Input: part model. Units: mm. Frame: model coordinates. A direction names the side the tool comes from. Coordinates: 2 decimals unless noted, no trailing zeros. Loops run counter-clockwise (first coordinate to the right, second up) from the corner with the lowest first, then second, coordinate; pieces in that order, holes last. Notation, with made-up numbers: (22.5, 86) - (56.5, 86) arc R21 cw to (56.5, 110) - close; hole circle Ø9 at (65, 2). An arc over 180 degrees is marked (long way). Use a Markdown table: item, result. Add a question column.
1. Section query C-C on z = 83.5. Return the cut outline in (x, y), then the cut area to 3 significant figures.
2. Ray query, L1, parallel to X at y = -7, z = 45; L2, parallel to X at y = -6.25, z = 29; L3, parallel to X at y = -3.25, z = 72.5. Return the intervals inside material, ascending. Write a range as [from, to].
3. Section query B-B on x = -112.5. Return the cut outline in (y, z), then the cut area to 3 significant figures.
4. Access query for faces 1 (the face through (-121.35, -4.06, 96.18)), 2 (the face through (8.5, -3.94, -32.05)), 3 (the face through (38, -4, -20)), 4 (the face through (35, -4, -16)), 5 (the face through (41, -4, -11)). Directions: +Z, -Z, +X, -X, +Y, -Y. A direction counts if a zero-diameter tool reaches every point of the face in a straight line with its end or side. Return the directions, or none.
5. Section query A-A on z = 55. Return the cut outline in (x, y).
6. Draft query along X for faces 6 (the face through (37.31, -3.94, -58.99)), 7 (the face through (-131.777, -3.944, 84.04)), 8 (the face through (-54.408, -3.944, 69.733)). Return one class per face: released by +X, released by -X, zero draft, split by the parting line, or undercut.
7. Contact query for flat-ended pins moving along their axis: P1, Ø3, axis at x = -110, y = -5.5, coming from the -Z side; P2, Ø23, axis at x = -58.49, z = 49.55, coming from the -Y side; P3, Ø2, axis at x = 41, y = -5, coming from the +Z side; P4, Ø4, axis at y = -4, z = -41, coming from the +X side. Output: stop coordinate, or through.
8. Section query D-D on y = -6. Return the cut outline in (x, z).
```python
from build123d import *

# Parameters (mm, degrees)
F0_R     = 10
F0_R_2   = 10.5
F1_DEPTH = 8
F2_R     = 15
F3_R     = 3.5


with BuildPart() as f1:
    # F0 (on Front) → F1 (new body)
    with BuildSketch(Plane.XZ):
        Polygon((-140.306121, 65.872547), (0, 0), (17.5, -66), (45.5, -66), (45.56593, -58.000272), (39.56593, -58.000272), (35, -60), (27, -60), (27, -12), (35, -12), (35, -20), (41, -20), (41, 0), (0, 44.189091), (-123.306754, 102.080578), align=None)
        with Locations((-58.485174, 49.552844)):
            Circle(F0_R, mode=Mode.SUBTRACT)
        with Locations((-113.249821, 75.264387)):
            Circle(F0_R_2, mode=Mode.SUBTRACT)
        with Locations((-85.641198, 62.30237)):
            Circle(F0_R, mode=Mode.SUBTRACT)
        with Locations((-31.329151, 36.803319)):
            Circle(F0_R, mode=Mode.SUBTRACT)
        with Locations((-4.173127, 24.053794)):
            Circle(F0_R, mode=Mode.SUBTRACT)
    extrude(amount=F1_DEPTH)

    # F2
    f2_edges = [f1.edges().sort_by_distance(p)[0] for p in [
        (-123.306754, -4, 102.080578),
        (-140.306121, -4, 65.872547),
    ]]
    fillet(f2_edges, radius=F2_R)

    # F3
    f3_edges = [f1.edges().sort_by_distance(p)[0] for p in [
        (0, -4, 0),
        (41, -4, 0),
        (0, -4, 44.189091),
        (45.56593, -4, -58.000272),
        (45.5, -4, -66),
        (17.5, -4, -66),
    ]]
    fillet(f3_edges, radius=F3_R)


solid = f1.part
```
Resolved:
| question | item | result |
|---|---|---|
| 1 | outline | (-132.03, -8) - (-119.76, -8) - (-119.76, 0) - (-132.03, 0) - close; (-106.74, -8) - (-83.73, -8) - (-83.73, 0) - (-106.74, 0) - close |
| 1 | area | 282 mm² |
| 2 | L1 | [-95.85, -67.39], [-49.58, -37.06], [-25.6, -1.73] |
| 2 | L2 | [-61.77, -37.58], [-25.08, -12.86], [4.52, 14.09] |
| 2 | L3 | [-135.34, -123.38], [-103.12, -60.3] |
| 3 | outline | (-8, 52.82) - (0, 52.82) - (0, 64.79) - (-8, 64.79) - close; (-8, 85.74) - (0, 85.74) - (0, 96.69) - (-8, 96.69) - close |
| 3 | area | 183 mm² |
| 4 | face 1 | +Z, +Y, -Y |
| 4 | face 2 | -Z, -X, +Y, -Y |
| 4 | face 3 | +X, +Y, -Y |
| 4 | face 4 | +Y, -Y |
| 4 | face 5 | +Z, +X, +Y, -Y |
| 5 | outline | (-117.15, -8) - (-92.47, -8) - (-92.47, 0) - (-117.15, 0) - close; (-78.81, -8) - (-66.87, -8) - (-66.87, 0) - (-78.81, 0) - close; (-50.1, -8) - (-23.03, -8) - (-23.03, 0) - (-50.1, 0) - close |
| 6 | face 6 | undercut |
| 6 | face 7 | released by -X |
| 6 | face 8 | released by +X |
| 7 | P1 | z = 50.94 |
| 7 | P2 | y = -8 |
| 7 | P3 | z = 1.08 |
| 7 | P4 | x = 27 |
| 8 | outline | (-133.93, 79.45) arc R15 ccw to (-126.73, 59.5) - (-1.48, 0.69) arc R3.5 cw to (0.42, -1.58) - (16.81, -63.4) arc R3.5 ccw to (20.19, -66) - (42.03, -66) arc R3.5 ccw to (45.53, -62.53) - (45.54, -61.53) arc R3.5 ccw to (42.04, -58) - (39.57, -58) - (35, -60) - (27, -60) - (27, -12) - (35, -12) - (35, -20) - (41, -20) - (41, -1.37) arc R3.5 ccw to (40.07, 1.01) - (0.46, 43.69) arc R3.5 ccw to (-0.62, 44.48) - (-109.73, 95.71) arc R15 ccw to (-129.68, 88.5) - close; hole circle Ø21 at (-113.25, 75.26); hole circle Ø20 at (-85.64, 62.3); hole circle Ø20 at (-58.49, 49.55); hole circle Ø20 at (-31.33, 36.8); hole circle Ø20 at (-4.17, 24.05) |
